```python
from build123d import *

# Parameters (mm, degrees)
SZKIC1_W                       = 12
SZKIC1_H                       = 66
DODANIE_WYCI_GNI_CIE1_DEPTH    = 41
OTW_R_GWINTOWANY_M5X0_81_D     = 4.2
OTW_R_GWINTOWANY_M5X0_81_DEPTH = 25
OTW_R_GWINTOWANY_M5X0_81_TIP   = 1.2618073
OTW_R_GWINTOWANY_M5X0_82_D     = 4.2
OTW_R_GWINTOWANY_M5X0_82_DEPTH = 25
OTW_R_GWINTOWANY_M5X0_82_TIP   = 1.2618073


with BuildPart() as part:
    # Szkic1 → Dodanie-wyciągnięcie1 (new body)
    with BuildSketch(Plane.XY):
        with Locations((-46, -22)):
            Rectangle(SZKIC1_W, SZKIC1_H)
    extrude(amount=DODANIE_WYCI_GNI_CIE1_DEPTH)

    # Otwór gwintowany M5x0.81
    with Locations(Plane(origin=(0, 0, 0), x_dir=(-1, 0, 0), z_dir=(0, 0, -1))):
        with Locations((46, -39), (46, -5)):
            Hole(OTW_R_GWINTOWANY_M5X0_81_D / 2, depth=OTW_R_GWINTOWANY_M5X0_81_DEPTH)
            with Locations((0, 0, -(OTW_R_GWINTOWANY_M5X0_81_DEPTH + OTW_R_GWINTOWANY_M5X0_81_TIP / 2))):  # 118° drill point
                Cone(0, OTW_R_GWINTOWANY_M5X0_81_D / 2, OTW_R_GWINTOWANY_M5X0_81_TIP, mode=Mode.SUBTRACT)

    # Otwór gwintowany M5x0.82
    with Locations(Plane.XY.offset(41)):
        with Locations((-46.43, -46.07), (-46.43, 1.07)):
            Hole(OTW_R_GWINTOWANY_M5X0_82_D / 2, depth=OTW_R_GWINTOWANY_M5X0_82_DEPTH)
            with Locations((0, 0, -(OTW_R_GWINTOWANY_M5X0_82_DEPTH + OTW_R_GWINTOWANY_M5X0_82_TIP / 2))):  # 118° drill point
                Cone(0, OTW_R_GWINTOWANY_M5X0_82_D / 2, OTW_R_GWINTOWANY_M5X0_82_TIP, mode=Mode.SUBTRACT)


solid = part.part
```
Read the model definition and answer for the solid it produces. Units are mm, in the model's axes. A direction names the side the tool comes from. Give positions to 0.01 mm unless a question says otherwise; leave off trailing zeros. Loops run counter-clockwise (first coordinate to the right, second up) from the corner with the lowest first, then second, coordinate; pieces in that order, holes last.
Item 1: For faces 1 (the cylindrical face through (-44.33, 1.16, 28.33)), 2 (the flat face through (-46, 11, 20)), 3 (the cylindrical face through (-45.031, -40.863, 12.675)), determine the directions among +Z, -Z, +X, -X, +Y, -Y from which every point of the face is accessible in a straight line to the end or side of a thin tool.
Item 2: Each of these flat-tipped pins is pushed along its axis until it touches: pin 1 Ø3.5 at (x, y) = (-46.43, 1.07) entering from +Z; pin 2 Ø2.5 at (x, y) = (-46, -39) entering from -Z. Where does it stop, or does it pass through?
Item 3: The part is cut by section A-A (z = 20). Write down the section's boundary in (x, y), and give its area (3 significant figures).
Item 4: The part is cut by section B-B (z = 30.5). Write down the section's boundary in (x, y).
Item 5: Find the intervals of material crossed by line 1 along Y through (x, z) = (-46.43, 35); line 2 along Y through (x, z) = (-46, 14); line 3 along X through (y, z) = (-5, 10.75), in increasing order.
Taken from the geometry:
1. face 1: +Z
1. face 2: +Z, -Z, +X, -X, +Y
1. face 3: -Z
2. pin 1: stops at z = 15.79
2. pin 2: stops at z = 25.51
3. outline: (-52, -55) - (-40, -55) - (-40, 11) - (-52, 11) - close; hole circle Ø4.2 at (-46.43, -46.07); hole circle Ø4.2 at (-46.43, 1.07); hole circle Ø4.2 at (-46, -39); hole circle Ø4.2 at (-46, -5)
3. area: 737 mm2
4. outline: (-52, -55) - (-40, -55) - (-40, 11) - (-52, 11) - close; hole circle Ø4.2 at (-46.43, -46.07); hole circle Ø4.2 at (-46.43, 1.07)
5. line 1: y = -55 to -48.17, -43.97 to -1.03, 3.17 to 11
5. line 2: y = -55 to -41.1, -36.9 to -7.1, -2.9 to 11
5. line 3: x = -52 to -48.1, -43.9 to -40
